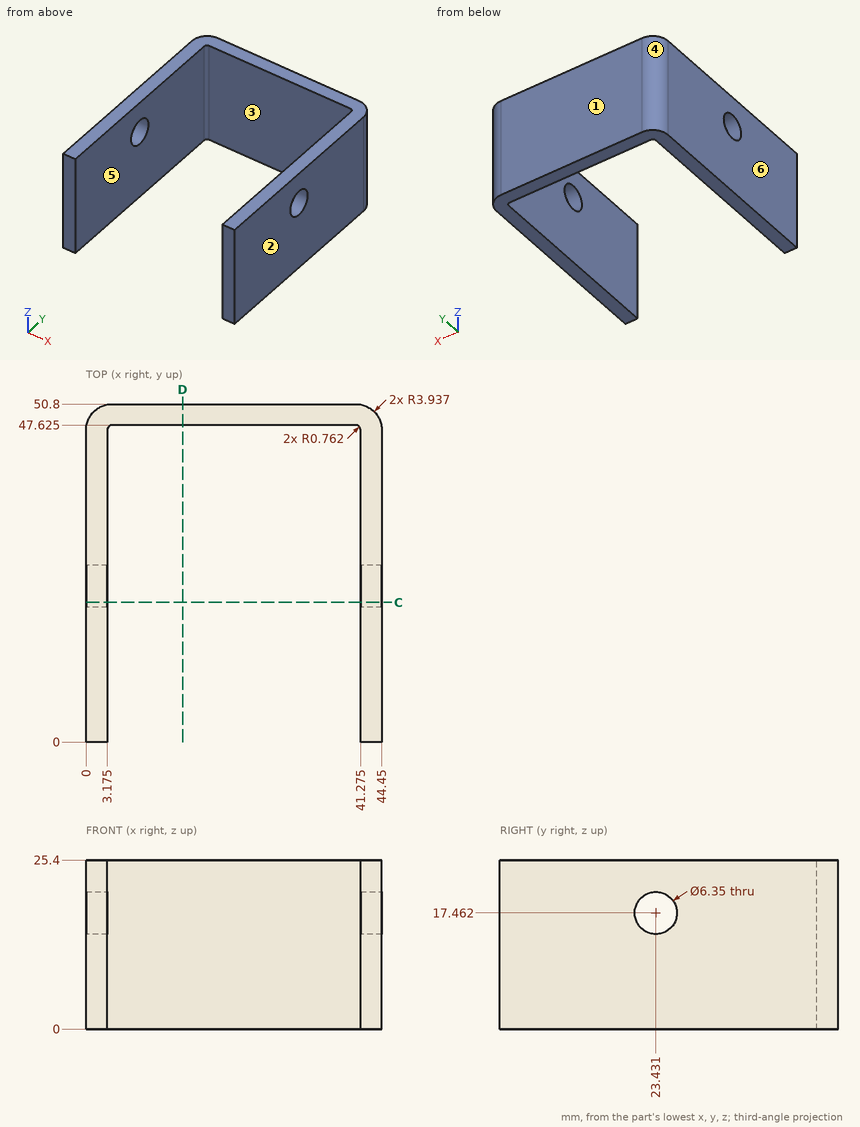
Job drawing, mm, ordinate dimensions from the low corner. One solid piece. A direction names the side the tool comes from. Coordinates: 2 decimals unless noted, no trailing zeros. Order: outer loops, then holes, each group sorted by start corner. A loop starts at its lowest first (then second) coordinate and runs counter-clockwise, first axis right, second up. Notation, with made-up numbers: (59.25, 85) - (64.25, 85) arc R37 cw to (64.25, 121) - close; hole circle Ø9 at (13, 31). An arc over 180 degrees is marked (long way). Return JSON: item names as keys, results as strings. Group by question number.
1) Probe line 1 (Y direction, x = 22.5, z = 22.75) (1 decimal); line 2 (Y direction, x = 2, z = 2.25). List the from-to ranges inside material, lowest first. Write a range as from..to.
2) Saw through at C-C, the plane y = 21. Count the separate pieces of the cut face and the enclosed holes in it, plus the area to 3 significant figures.
3) Tool access for the marked faces 5 and 6: list every direction of +Z, -Z, +X, -X, +Y, -Y with a clear straight run to the whole face (end or side of a thin tool).
4) Mould opens along X. For the marked faces 1, 2, 3 and 4 say: released by +X, released by -X, zero draft, split by the parting line, or undercut.
5) Flat gauge pins, fed straight in: P1, Ø8, axis at x = 15.5, z = 17, coming from the -Y side (1 decimal); P2, Ø5, axis at x = 38.5, z = 16, coming from the -Y side. Where does each tip first touch, or does it go through?
6) Saw through at D-D, the plane x = 14.5. Write the cut outline in (y, z) (1 decimal).
Values found:
{
 "1": {"line 1": "y = 47.6..50.8", "line 2": "y = 0..50.29"},
 "2": {"separate pieces": "4", "enclosed holes": "0", "area": "135 mm²"},
 "3": {"face 5": "+Z, -Z, -Y", "face 6": "+Z, -Z, -X, +Y, -Y"},
 "4": {"face 1": "zero draft", "face 2": "released by +X", "face 3": "undercut", "face 4": "released by -X"},
 "5": {"P1": "stops at y = 47.6", "P2": "stops at y = 47.45"},
 "6": {"outline": "(47.6, 0) - (50.8, 0) - (50.8, 25.4) - (47.6, 25.4) - close"}
}
